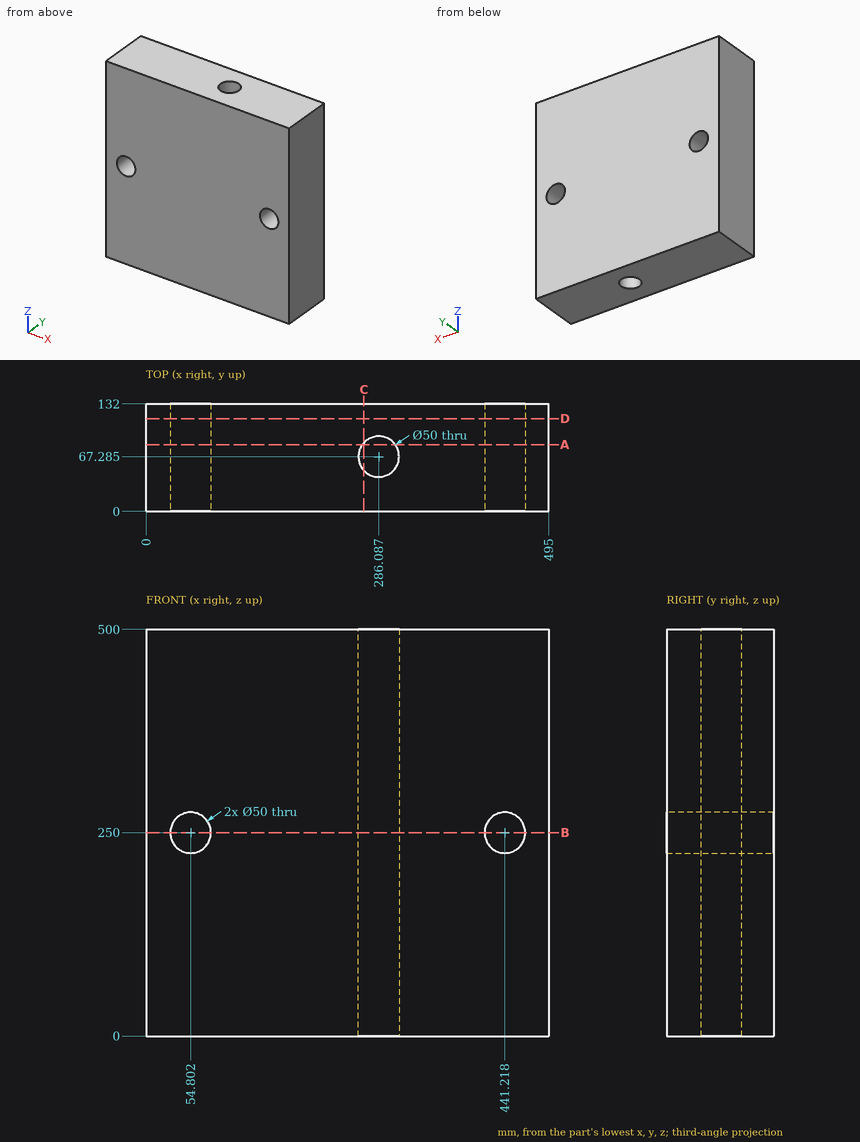
Verification items for this drawing (mm, ordinates from the low corner). Coordinates: 2 decimals unless noted, no trailing zeros. Write each loop counter-clockwise with the first axis right and the second up, starting at its lowest first coordinate (ties: lowest second). Pieces come first, ordered by that corner, then holes. Notation, with made-up numbers: M 72,-16 L 82,-16 A19 cw 82,-9 Z; hole C 38,-21.5 d3. An arc over 180 degrees is marked long. Answer as a JSON object with one key per item and string values.
1. Section check A-A, the plane y = 82. Enter the section's corners in (x, z), plus the area to 3 significant figures.
Answers below:
{"outline": "M 0,0 L 265.88,0 L 265.88,500 L 0,500 Z; M 306.3,0 L 495,0 L 495,500 L 306.3,500 Z; hole C 54.8,250 d50; hole C 441.22,250 d50", "area": "223,000 mm²"}
2. Scan lines: L1, parallel to X at y = 102.5, z = 250; L2, parallel to X at y = 90, z = 250 (1 decimal); L3, parallel to X at y = 54.5, z = 253.5 (1 decimal). Record each from-to range of solid material in increasing order.
Answers below:
{"L1": "x = 0 to 29.8, 79.8 to 416.22, 466.22 to 495", "L2": "x = 0 to 29.8, 79.8 to 275.6, 296.5 to 416.2, 466.2 to 495", "L3": "x = 0 to 30, 79.6 to 264.6, 307.6 to 416.5, 466 to 495"}
3. Section check B-B, the plane z = 250. Enter the section's corners in (x, y) (1 decimal), plus the area to 3 significant figures.
Answers below:
{"outline": "M 0,0 L 29.8,0 L 29.8,132 L 0,132 Z; M 79.8,0 L 416.2,0 L 416.2,132 L 79.8,132 Z; M 466.2,0 L 495,0 L 495,132 L 466.2,132 Z; hole C 286.1,67.3 d50", "area": "50,200 mm²"}
4. Section check D-D, the plane y = 114. Enter the section's corners in (x, z).
Answers below:
{"outline": "M 0,0 L 495,0 L 495,500 L 0,500 Z; hole C 54.8,250 d50; hole C 441.22,250 d50"}
5. Go/stop test with a flat-tipped pin: pin 1 Ø2 at (x, z) = (115, 400.5) entering from -Y. Record where the tip stops, or that it passes through.
Answers below:
{"pin 1": "stops at y = 0"}
6. Section check C-C, the plane x = 268. Enter the section's corners in (y, z), plus the area to 3 significant figures.
Answers below:
{"outline": "M 0,0 L 50.03,0 L 50.03,500 L 0,500 Z; M 84.54,0 L 132,0 L 132,500 L 84.54,500 Z", "area": "48,700 mm²"}
